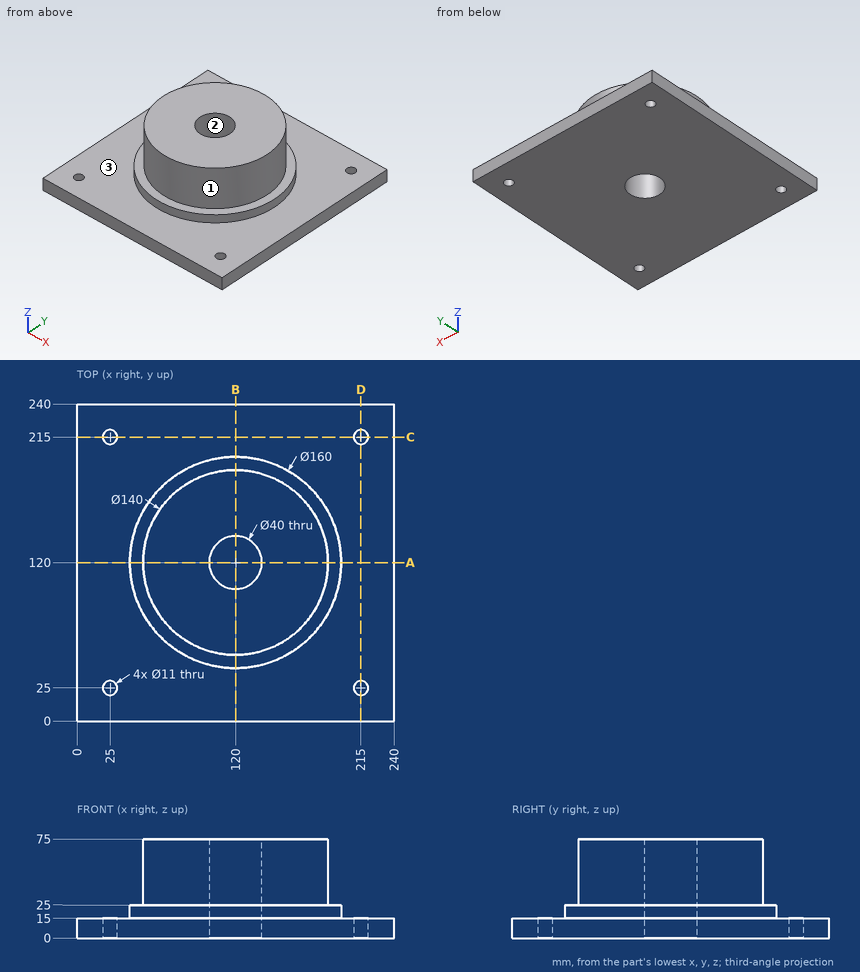
Here's the drawing with two shaded views (mm, measured from the low corner). I have some questions. Coordinates: 2 decimals unless noted, no trailing zeros. Write each loop counter-clockwise with the first axis right and the second up, starting at its lowest first coordinate (ties: lowest second). Pieces come first, ordered by that corner, then holes. Notation, with made-up numbers: M -28,5.25 L 8,5.25 A27 ccw 8,38.25 Z; hole C -32,-6 d2. An arc over 180 degrees is marked long. Use one line per item in the form item = value.
Q1. For P1, Ø8, axis at y = 44.5, z = 22.5, coming from the +X side; P2, Ø8, axis at x = 136.5, y = 215, coming from the +Z side; P3, Ø2, axis at x = 124.5, z = 39, coming from the +Y side, each with a flat end and sliding along its axis, tell me the tip position at first contact or that it passes through.
Model answer:
P1 = 155.89
P2 = 15
P3 = 189.91
Q2. I need wall thicknesses on line 1 along Y through (x, z) = (25, 5.25); line 2 along Y through (x, z) = (120, 46). Which ranges of each line are inside material? Lowest first, please. Write a range as from..to.
Model answer:
line_1 = 0..19.5, 30.5..209.5, 220.5..240
line_2 = 50..100, 140..190
Q3. If we section it at A-A (y = 120): Write out the boundary of the cut face in (x, z), then the cut area to 3 significant figures.
Model answer:
outline = M 0,0 L 100,0 L 100,75 L 50,75 L 50,25 L 40,25 L 40,15 L 0,15 Z; M 140,0 L 240,0 L 240,15 L 200,15 L 200,25 L 190,25 L 190,75 L 140,75 Z
area = 9,200 mm^2
Q4. We'd pull the mould along Y, two halves only. Please class the marked faces 1, 2 and 3: +Y half, -Y half, draft (parallel to the pull), parting line (faces both ways), or undercut.
Model answer:
face_1 = parting line
face_2 = undercut
face_3 = draft
Q5. If we section it at C-C (y = 215): Write out the boundary of the cut face in (x, z), then the cut area to 3 significant figures.
Model answer:
outline = M 0,0 L 19.5,0 L 19.5,15 L 0,15 Z; M 30.5,0 L 209.5,0 L 209.5,15 L 30.5,15 Z; M 220.5,0 L 240,0 L 240,15 L 220.5,15 Z
area = 3,270 mm^2
